```python
from build123d import *


with BuildPart() as part:
    # Эскиз1 → Повернуть1 (revolve)
    with BuildSketch(Plane(origin=(0, 0, 0), x_dir=(0, 0, -1), z_dir=(1, 0, 0))):
        with BuildLine():
            Line((2.5, 3.5), (1.5, 3.5))
            Line((1.5, 3.5), (1.5, -3.5))
            Line((1.5, -3.5), (2.5, -3.5))
            Line((2.5, -3.5), (1.708705964, -2.708705964))
            ThreePointArc((1.708705964, -2.708705964), (1.621467661, -2.477147118), (1.737901046, -2.258804984))
            ThreePointArc((1.737901046, -2.258804984), (2.85, 0), (1.737901046, 2.258804984))
            ThreePointArc((1.737901046, 2.258804984), (1.621467661, 2.477147118), (1.708705964, 2.708705964))
            Line((1.708705964, 2.708705964), (2.5, 3.5))
        make_face()
    revolve(axis=Axis((0, 0, 0), (0, -1, 0)))


solid = part.part
```
Source: CAD feature listing. Evaluate the final solid. Frame: model axes, mm. A direction names the side the tool comes from. Round coordinates to 2 decimals unless told otherwise and drop trailing zeros. Loops run counter-clockwise (first coordinate to the right, second up) from the corner with the lowest first, then second, coordinate; pieces in that order, holes last. Notation, with made-up numbers: M -36,20.25 L -18,20.25 A21 cw -18,34.25 Z; hole C -12.75,-24 d7. An arc over 180 degrees is marked long. Use a Markdown table: item, result. Add a question column.
1. Cut plane B-B, the plane x = 0. Output: boundary loops of the cut face in (y, z).
2. Pull-direction query (Y, two-part tool) for faces 1 (the cylindrical face through (0.07, -0.05, 1.5)), 2 (the flat face through (0, -3.5, 2)), 3 (the conical face through (2, -3, 0)); classes: +Y half, -Y half, draft (parallel to the pull), parting line (faces both ways), or undercut.
3. Set-up query: faces 4 (the conical face through (0, 3, 2)), 5 (the flat face through (0, 3.5, -2)). Return all of +Z, -Z, +X, -X, +Y, -Y with unobstructed straight access to the full face (end or side cutting, diameter ignored); none if empty.
4. Contact query for flat-ended pins moving along their axis: pin 1 (3 mm diameter, centred on x = 1, z = -0.5, fed in from -Y); pin 2 (1.5 mm diameter, centred on y = 1.5, z = -1, fed in from +X). Output: stop coordinate, or through.
5. Cut plane A-A, the plane z = 0. Output: boundary loops of the cut face in (x, y).
6. Cut plane C-C, the plane y = -2.5. Output: boundary loops of the cut face in (x, z), and give its area (3 significant figures).
7. Ray query, line 1 along Y through (x, z) = (0.95, -1.55); line 2 along X through (y, z) = (-1.75, 0); line 3 along Z through (x, y) = (0.8, 1.5). Return the intervals inside material, ascending. Write a range as [from, to].
8. Cut plane D-D, the plane z = 1.9. State how many separate pieces and enclosed holes the cut face has, and give its area (3 significant figures).
Solution:
| question | item | result |
|---|---|---|
| 1 | outline | M -3.5,-2.5 L -2.71,-1.71 A0.3 cw -2.26,-1.74 A2.85 ccw 2.26,-1.74 A0.3 cw 2.71,-1.71 L 3.5,-2.5 L 3.5,-1.5 L -3.5,-1.5 Z; M -3.5,1.5 L 3.5,1.5 L 3.5,2.5 L 2.71,1.71 A0.3 cw 2.26,1.74 A2.85 ccw -2.26,1.74 A0.3 cw -2.71,1.71 L -3.5,2.5 Z |
| 2 | face 1 | draft |
| 2 | face 2 | -Y half |
| 2 | face 3 | undercut |
| 3 | face 4 | none |
| 3 | face 5 | +Z, -Z, +X, -X, +Y |
| 4 | pin 1 | stops at y = -3.5 |
| 4 | pin 2 | stops at x = 2.65 |
| 5 | outline | M -2.5,-3.5 L -1.5,-3.5 L -1.5,3.5 L -2.5,3.5 L -1.71,2.71 A0.3 cw -1.74,2.26 A2.85 ccw -1.74,-2.26 A0.3 cw -1.71,-2.71 Z; M 1.5,-3.5 L 2.5,-3.5 L 1.71,-2.71 A0.3 cw 1.74,-2.26 A2.85 ccw 1.74,2.26 A0.3 cw 1.71,2.71 L 2.5,3.5 L 1.5,3.5 Z |
| 6 | outline | C 0,0 d3.24; hole C 0,0 d3 |
| 6 | area | 1.18 mm2 |
| 7 | line 1 | y = [-3.5, -2.82], [-2.19, 2.19], [2.82, 3.5] |
| 7 | line 2 | x = [-2.25, -1.5], [1.5, 2.25] |
| 7 | line 3 | z = [-2.29, -1.27], [1.27, 2.29] |
| 8 | separate pieces | 3 |
| 8 | enclosed holes | 0 |
| 8 | area | 16.7 mm2 |
